The drawing under review shows one solid part. Ordinate dimensions are in mm from its lowest x, y, z. A direction names the side the tool comes from. Coordinates: 2 decimals unless noted, no trailing zeros. Loops run counter-clockwise (first coordinate to the right, second up) from the corner with the lowest first, then second, coordinate; pieces in that order, holes last. Notation, with made-up numbers: M -5.75,84 L 27.25,84 A19 cw 27.25,121 Z; hole C 45,75 d7. An arc over 180 degrees is marked long. Use one line per item in the form item = value.
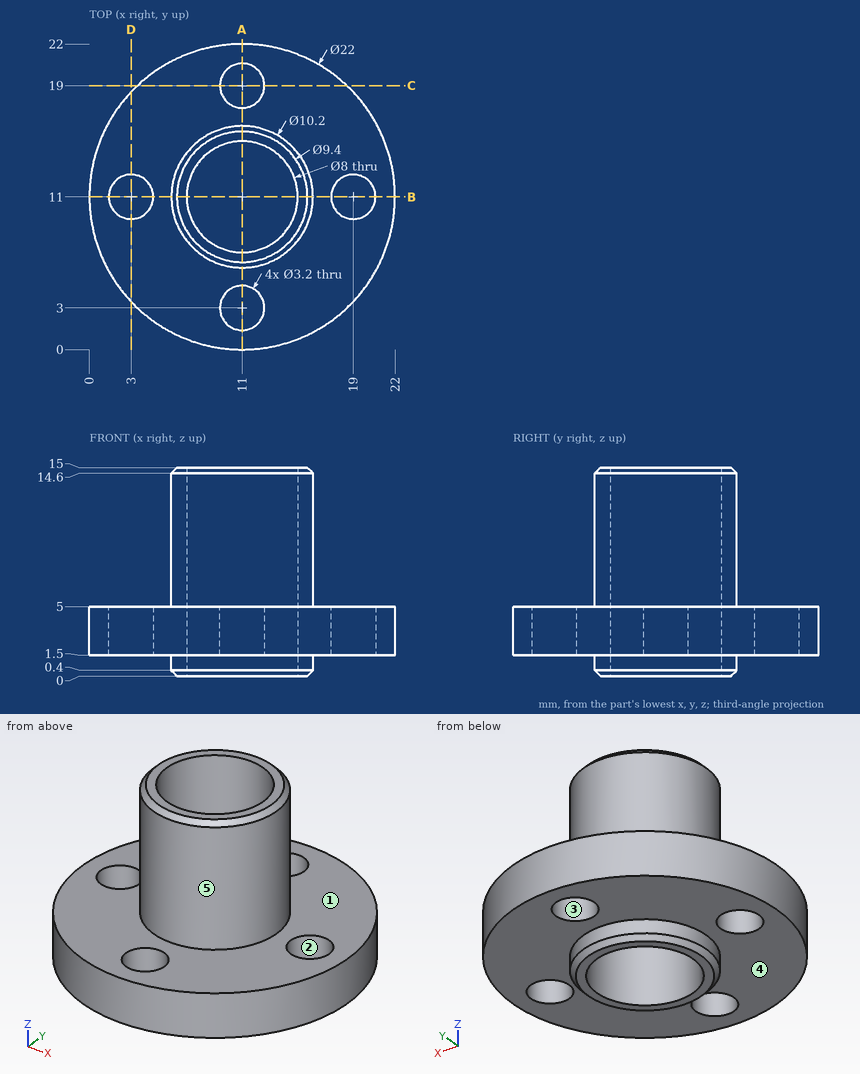
1. Wall thickness on line 1 along Y through (x, z) = (11, 3.95); line 2 along Y through (x, z) = (11, 9.25); line 3 along Z through (x, y) = (11.25, 16.75): over which ranges is each line inside the solid? List them lowest first. Write a range as from..to.
Computed values:
line_1 = 0..1.4, 4.6..7, 15..17.4, 20.6..22
line_2 = 5.9..7, 15..16.1
line_3 = 1.5..5
2. Draft analysis for pull direction Y (two halves, no side actions). For the marked faces 3, 4 and 5, state which applies: +Y half, -Y half, draft (parallel to the pull), parting line (faces both ways), or undercut.
Computed values:
face_3 = undercut
face_4 = draft
face_5 = parting line
3. For pin 1 Ø3.5 at (x, y) = (3, 11) entering from -Z; pin 2 Ø1.9 at (x, y) = (11, 19) entering from +Z; pin 3 Ø3 at (y, z) = (8.5, 6) entering from -X; pin 4 Ø5 at (y, z) = (3, 2.5) entering from -X, all flat-tipped, find the tip position at first contact; note any pin that passes through.
Computed values:
pin_1 = 1.5
pin_2 = through
pin_3 = 0.09
pin_4 = 1.47
4. Consider section C-C on y = 19. Write out the cut boundary in (x, z), plus the area to 3 significant figures.
Computed values:
outline = M 3.45,1.5 L 9.4,1.5 L 9.4,5 L 3.45,5 Z; M 12.6,1.5 L 18.55,1.5 L 18.55,5 L 12.6,5 Z
area = 41.6 mm2
5. Tool access review of the marked faces 1 and 2: name each direction out of +Z, -Z, +X, -X, +Y, -Y from which nothing blocks a thin tool from reaching the whole face with its end or side.
Computed values:
face_1 = +Z
face_2 = +Z, -Z
6. Consider section A-A on x = 11. Write out the cut boundary in (y, z).
Computed values:
outline = M 0,1.5 L 1.4,1.5 L 1.4,5 L 0,5 Z; M 4.6,1.5 L 5.9,1.5 L 5.9,0.4 L 6.3,0 L 7,0 L 7,15 L 6.3,15 L 5.9,14.6 L 5.9,5 L 4.6,5 Z; M 15,0 L 15.7,0 L 16.1,0.4 L 16.1,1.5 L 17.4,1.5 L 17.4,5 L 16.1,5 L 16.1,14.6 L 15.7,15 L 15,15 Z; M 20.6,1.5 L 22,1.5 L 22,5 L 20.6,5 Z
